Geometry: final body of the model. Coordinates: model frame, mm. Round coordinates to 2 decimals unless told otherwise and drop trailing zeros. Write each loop counter-clockwise with the first axis right and the second up, starting at its lowest first coordinate (ties: lowest second). Pieces come first, ordered by that corner, then holes. Notation, with made-up numbers: (47, -3) - (104, -3) arc R25 cw to (104, 19) - close; hole circle Ø3 at (86, -13). An arc over 180 degrees is marked (long way). Write each question's results on one line, items separated by ' | '.
from build123d import *

# Parameters (mm, degrees)
SKETCH1_W           = 229.859874896
SKETCH1_H           = 6.35
BOSS_EXTRUDE1_DEPTH = 152.4
SKETCH2_W           = 25.4
SKETCH2_H           = 6.35
BOSS_EXTRUDE2_DEPTH = 6.35
LPATTERN1_COUNT     = 4
LPATTERN1_PITCH     = 50.8
SKETCH3_W           = 25.4
SKETCH3_H           = 6.35
BOSS_EXTRUDE3_DEPTH = 6.35
LPATTERN2_COUNT     = 4
LPATTERN2_PITCH     = 50.8
CUT_EXTRUDE1_DEPTH  = 6.35
SKETCH5_W           = 6.35
SKETCH5_H           = 12.7
CUT_EXTRUDE2_DEPTH  = 212.329778686
SKETCH6_R           = 2.0955
CUT_EXTRUDE3_DEPTH  = 212.329778686


with BuildPart() as part:
    # Sketch1 → Boss-Extrude1 (new body)
    with BuildSketch(Plane.XY):
        with Locations((-24.419947229, 152.4)):
            Rectangle(SKETCH1_W, SKETCH1_H)
    extrude(amount=BOSS_EXTRUDE1_DEPTH)

    # Sketch2 → Boss-Extrude2 (add)
    with BuildSketch(Plane(origin=(0, 155.575, 0), x_dir=(1, 0, 0), z_dir=(0, 1, 0))):
        with Locations((52.409990219, 3.175)):
            Rectangle(SKETCH2_W, SKETCH2_H)
    boss_extrude2 = extrude(amount=-BOSS_EXTRUDE2_DEPTH)

    # LPattern1: Boss-Extrude2 ×4
    with Locations(*[(-i * LPATTERN1_PITCH, 0, 0) for i in range(1, LPATTERN1_COUNT)]):
        add(boss_extrude2)

    # Sketch3 → Boss-Extrude3 (add)
    with BuildSketch(Plane.XY.offset(152.4)):
        with Locations((52.409990219, 152.4)):
            Rectangle(SKETCH3_W, SKETCH3_H)
    boss_extrude3 = extrude(amount=BOSS_EXTRUDE3_DEPTH)

    # LPattern2: Boss-Extrude3 ×4
    with Locations(*[(-i * LPATTERN2_PITCH, 0, 0) for i in range(1, LPATTERN2_COUNT)]):
        add(boss_extrude3)

    # Sketch4 → Cut-Extrude1 (cut)
    with BuildSketch(Plane(origin=(0, 155.575, 0), x_dir=(1, 0, 0), z_dir=(0, 1, 0))):
        Polygon((-123.886347229, 0), (-128.153547229, 0), (-128.153547229, -8.763), (-130.464947229, -8.763), (-130.464947229, -11.938), (-128.153547229, -11.938), (-128.153547229, -15.24), (-123.886347229, -15.24), (-123.886347229, -11.938), (-121.574947229, -11.938), (-121.574947229, -8.763), (-123.886347229, -8.763), align=None)
        Polygon((-21.656409781, 0), (-25.923609781, 0), (-25.923609781, -8.763), (-28.235009781, -8.763), (-28.235009781, -11.938), (-25.923609781, -11.938), (-25.923609781, -15.24), (-21.656409781, -15.24), (-21.656409781, -11.938), (-19.345009781, -11.938), (-19.345009781, -8.763), (-21.656409781, -8.763), align=None)
        Polygon((79.943590219, 0), (75.676390219, 0), (75.676390219, -8.763), (73.364990219, -8.763), (73.364990219, -11.938), (75.676390219, -11.938), (75.676390219, -15.24), (79.943590219, -15.24), (79.943590219, -11.938), (82.254990219, -11.938), (82.254990219, -8.763), (79.943590219, -8.763), align=None)
        Polygon((-128.153547229, -152.4), (-123.886347229, -152.4), (-123.886347229, -143.637), (-121.574947229, -143.637), (-121.574947229, -140.462), (-123.886347229, -140.462), (-123.886347229, -137.16), (-128.153547229, -137.16), (-128.153547229, -140.462), (-130.464947229, -140.462), (-130.464947229, -143.637), (-128.153547229, -143.637), align=None)
        Polygon((-25.923609781, -152.4), (-21.656409781, -152.4), (-21.656409781, -143.637), (-19.345009781, -143.637), (-19.345009781, -140.462), (-21.656409781, -140.462), (-21.656409781, -137.16), (-25.923609781, -137.16), (-25.923609781, -140.462), (-28.235009781, -140.462), (-28.235009781, -143.637), (-25.923609781, -143.637), align=None)
        Polygon((75.676390219, -152.4), (79.943590219, -152.4), (79.943590219, -143.637), (82.254990219, -143.637), (82.254990219, -140.462), (79.943590219, -140.462), (79.943590219, -137.16), (75.676390219, -137.16), (75.676390219, -140.462), (73.364990219, -140.462), (73.364990219, -143.637), (75.676390219, -143.637), align=None)
    extrude(amount=-CUT_EXTRUDE1_DEPTH, mode=Mode.SUBTRACT)

    # Sketch5 → Cut-Extrude2 (cut, through all)
    with BuildSketch(Plane(origin=(0, 155.575, 0), x_dir=(1, 0, 0), z_dir=(0, 1, 0))):
        with Locations((-129.824884677, -44.45)):
            Rectangle(SKETCH5_W, SKETCH5_H)
        with Locations((-129.824884677, -69.85)):
            Rectangle(SKETCH5_W, SKETCH5_H)
    extrude(amount=-CUT_EXTRUDE2_DEPTH, mode=Mode.SUBTRACT)

    # Sketch6 → Cut-Extrude3 (cut, through all)
    with BuildSketch(Plane(origin=(0, 155.575, 0), x_dir=(1, 0, 0), z_dir=(0, 1, 0))):
        with Locations(Location((-129.824884677, -89.98, 0), (0, 0, 270))):
            Circle(SKETCH6_R)
        with Locations(Location((-129.824884677, -24.32, 0), (0, 0, 270))):
            Circle(SKETCH6_R)
    extrude(amount=-CUT_EXTRUDE3_DEPTH, mode=Mode.SUBTRACT)


solid = part.part
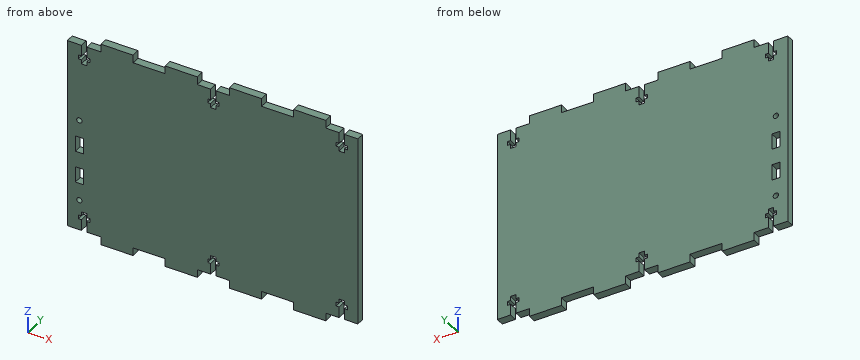
Q1. Section query A-A, the plane x = -33.5. Return loops of the section in (y, z) (3 decimals).
Answer block:
outline: (149.225, 0) - (155.575, 0) - (155.575, 152.4) - (149.225, 152.4) - close
Q2. Section query B-B, the plane y = 150.5. Give the number of separate pieces and of enclosed holes in the cut face, plus the area to 3 significant figures.
Answer block:
separate pieces: 1 | enclosed holes: 4 | area: 35,700 mm2
Q3. Ray query, line 1 along Z through (x, y) = (-127.5, 150.75); line 2 along Z through (x, y) = (81, 152.75); line 3 along X through (y, z) = (152.25, 24.32). Return the intervals inside material, ascending.
Answer block:
line 1: 15.24 to 38.1, 50.8 to 63.5, 76.2 to 137.16 | line 2: 0 to 8.76, 11.94 to 140.46, 143.64 to 152.4 | line 3: -139.35 to -131.92, -127.73 to 90.51
Q4. Pin query (flat end, axial travel): pin 1 (1.9 mm diameter, centred on x = -130, y = 151.5, fed in from -Z); pin 2 (1.8 mm diameter, centred on x = 81, y = 153, fed in from +Z); pin 3 (1.3 mm diameter, centred on x = -24, y = 151, fed in from -Z). Return the tip coordinate at first contact, or that it passes through.
Answer block:
pin 1: z = 0 | pin 2: z = 152.4 | pin 3: z = 15.24
